```python
from build123d import *

# Parameters (mm, degrees)
F0_R            = 32.0294
F0_R_2          = 2.15265
F0_R_3          = 14.2875
F1_DEPTH        = 3.175
F3_DEPTH        = 3.175
F3_COPIES_COUNT = 4


# Not quite as in the source:
# - a pattern or mirror of a feature is missing from the dataset's text; its kind, count and spacing are read off the source's solid


with BuildPart() as f1:
    # F0 (on Top) → F1 (new body)
    with BuildSketch(Plane.XY):
        Circle(F0_R)
        with Locations((-14.0316501892, -14.0316501892)):
            Circle(F0_R_2, mode=Mode.SUBTRACT)
        with Locations((14.0316501892, -14.0316501892)):
            Circle(F0_R_2, mode=Mode.SUBTRACT)
        with Locations((-14.0316501892, 14.0316501892)):
            Circle(F0_R_2, mode=Mode.SUBTRACT)
        Circle(F0_R_3, mode=Mode.SUBTRACT)
        with Locations((14.0316501892, 14.0316501892)):
            Circle(F0_R_2, mode=Mode.SUBTRACT)
    extrude(amount=F1_DEPTH)

    # F2 (on face) → F3 (cut, through all)
    with BuildSketch(Plane.XY.offset(3.175)):
        with BuildLine():
            ThreePointArc((-12.0590655259, 19.2259570543), (-9.8169566913, 17.6521850643), (-8.599282572, 15.1983961488))
            ThreePointArc((-8.599282572, 15.1983961488), (0, 17.4625), (8.599282572, 15.1983961488))
            ThreePointArc((8.599282572, 15.1983961488), (9.8169566913, 17.6521850643), (12.0590655259, 19.2259570543))
            ThreePointArc((12.0590655259, 19.2259570543), (0, 22.6949), (-12.0590655259, 19.2259570543))
        make_face()
    f3 = extrude(amount=-F3_DEPTH, mode=Mode.SUBTRACT)

    # F3_copies: F3 ×4 about axis
    f3_copies_axis = Axis((0, 0, 0), (0, 0, 1))
    for i in range(1, F3_COPIES_COUNT):
        add(f3.rotate(f3_copies_axis, i * 360 / F3_COPIES_COUNT), mode=Mode.SUBTRACT)


solid = f1.part
```
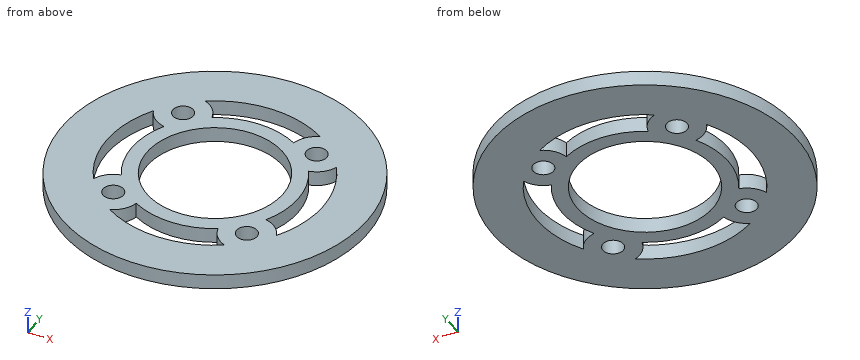
Could you check a few things on this model? Use its own coordinates, in mm. Round coordinates to 2 decimals unless told otherwise and drop trailing zeros. Write each loop counter-clockwise with the first axis right and the second up, starting at its lowest first coordinate (ties: lowest second). Pieces come first, ordered by that corner, then holes.
(1) Suppose I cut it at C-C on z = 1.3. State how many separate pieces and enclosed holes the cut face has, and give its area (3 significant figures).
Findings below:
separate pieces: 1
enclosed holes: 9
area: 2,090 mm2
(2) For pin 1 (1 mm diameter, centred on y = -13.5, z = 1.5, fed in from -X); pin 2 (1.5 mm diameter, centred on x = 8, z = 1, fed in from +Y), each with a flat end and sliding along its axis, tell me the tip position at first contact or that it passes through.
Findings below:
pin 1: stops at x = -29.27
pin 2: stops at y = 31.2
(3) Suppose I cut it at D-D on y = -18.5. Write out the boundary of the cut face in (x, z) (3 decimals).
Findings below:
outline: (-26.146, 0) - (-10.729, 0) - (-10.729, 3.175) - (-26.146, 3.175) - close; (10.729, 0) - (26.146, 0) - (26.146, 3.175) - (10.729, 3.175) - close
(4) If I drill on probe 1 along Y at (x, z) = (0, 1.6); probe 2 along X at (y, z) = (-3.5, 0.65); probe 3 along Y at (x, z) = (6, 1.5), over which ranges is the centre line in solid material (lowest first)?
Findings below:
probe 1: y = -32.03 to -22.69, -17.46 to -14.29, 14.29 to 17.46, 22.69 to 32.03
probe 2: x = -31.84 to -22.42, -17.11 to -13.85, 13.85 to 17.11, 22.42 to 31.84
probe 3: y = -31.46 to -21.89, -16.4 to -12.97, 12.97 to 16.4, 21.89 to 31.46
(5) Suppose I cut it at A-A on y = 0. Write out the boundary of the cut face in (x, z) (1 decimal), and give its area (3 significant figures).
Findings below:
outline: (-32, 0) - (-22.7, 0) - (-22.7, 3.2) - (-32, 3.2) - close; (-17.5, 0) - (-14.3, 0) - (-14.3, 3.2) - (-17.5, 3.2) - close; (14.3, 0) - (17.5, 0) - (17.5, 3.2) - (14.3, 3.2) - close; (22.7, 0) - (32, 0) - (32, 3.2) - (22.7, 3.2) - close
area: 79.4 mm2
